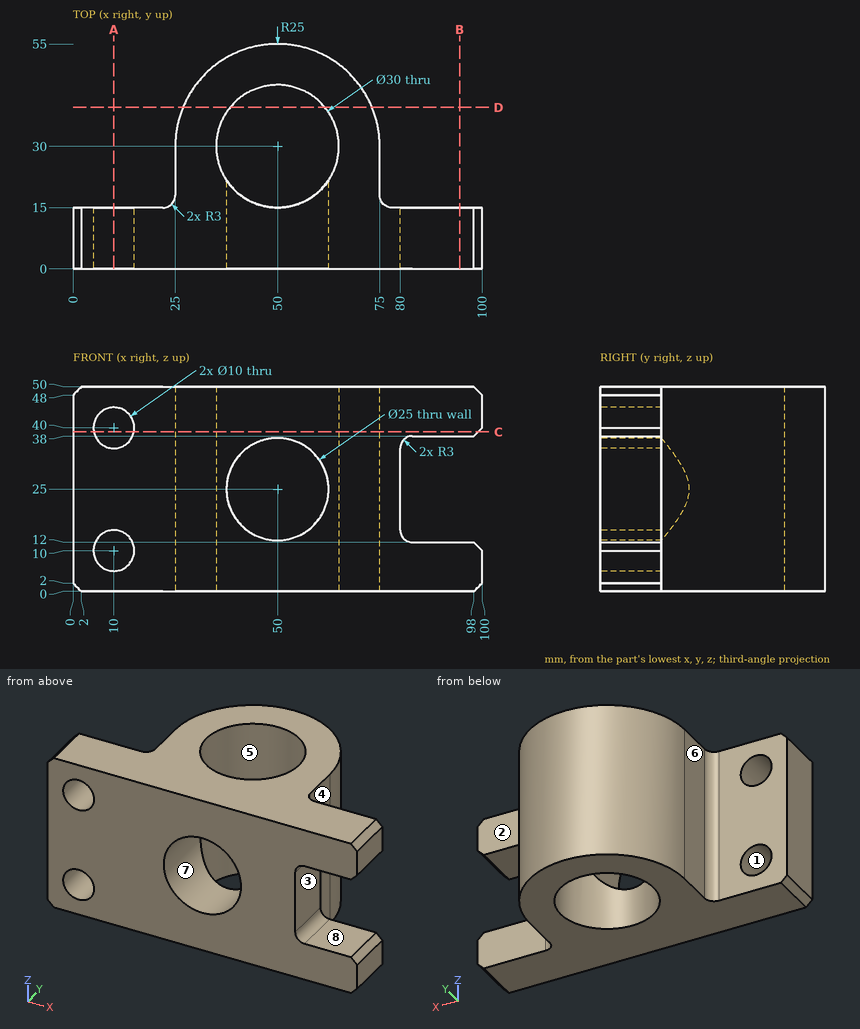
Here's the drawing with two shaded views (mm, measured from the low corner). I have some questions. A direction names the side the tool comes from. Give positions to 0.01 mm unless a question says otherwise; leave off trailing zeros. Loops run counter-clockwise (first coordinate to the right, second up) from the corner with the lowest first, then second, coordinate; pieces in that order, holes last. Notation, with made-up numbers: M 87.5,33 L 99.5,33 A19 cw 99.5,58 Z; hole C 47,76 d1. An arc over 180 degrees is marked long. One line per item, written item: value. Start each with the question number.
1) Thinking about a two-plate mould opening in X: for the marked faces 1, 2 and 3, which applies, +X half, -X half, draft (parallel to the pull), parting line (faces both ways), or undercut?
2) If we section it at B-B, the plane x = 94.5: Write out the boundary of the cut face in (y, z).
3) If we section it at A-A, the plane x = 10: Write out the boundary of the cut face in (y, z).
4) I'm going to push flat-ended pins straight in: pin 1 (2 mm diameter, centred on x = 52.5, z = 15, fed in from -Y); pin 2 (8 mm diameter, centred on x = 28, z = 17.5, fed in from +Y); pin 3 (12 mm diameter, centred on y = 5, z = 21.5, fed in from +X). Where does each tip first touch, or does it pass through?
5) On a 3-axis mill with a long thin cutter (end or side, diameter ignored), from which of +Z, -Z, +X, -X, +Y, -Y can I reach the whole of each face in a straight line? I mean the marked faces 4, 5, 6, 7 and 8. Say none if no direction works.
6) If we section it at D-D, the plane y = 39.5: Write out the boundary of the cut face in (x, z).
7) If we section it at C-C, the plane z = 39: Write out the boundary of the cut face in (x, y), and give its area (3 significant figures).
8) If I drill on line 1 (Z direction, x = 10, y = 4.25); line 2 (Z direction, x = 42.5, y = 12); line 3 (Y direction, x = 16.5, z = 37.5), over which ranges is the centre line in solid material (lowest first)? Write a range as [from, to].
Completed:
1. face 1: undercut
1. face 2: draft
1. face 3: +X half
2. outline: M 0,0 L 15,0 L 15,12 L 0,12 Z; M 0,38 L 15,38 L 15,50 L 0,50 Z
3. outline: M 0,0 L 15,0 L 15,5 L 0,5 Z; M 0,15 L 15,15 L 15,35 L 0,35 Z; M 0,45 L 15,45 L 15,50 L 0,50 Z
4. pin 1: stops at y = 44.59
4. pin 2: stops at y = 47.35
4. pin 3: stops at x = 80
5. face 4: +Z, -Z, +X, +Y
5. face 5: +Z, -Z
5. face 6: +Z, -Z, -X, +Y
5. face 7: -Y
5. face 8: +X, +Y, -Y
6. outline: M 26.88,0 L 38.39,0 L 38.39,50 L 26.88,50 Z; M 61.61,0 L 73.12,0 L 73.12,50 L 61.61,50 Z
7. outline: M 0,0 L 5.1,0 L 5.1,15 L 0,15 Z; M 14.9,0 L 99,0 L 99,15 L 78,15 A3 cw 75,18 L 75,30 A25 ccw 25,30 L 25,18 A3 cw 22,15 L 14.9,15 Z; hole C 50,30 d30
7. area: 2,370 mm^2
8. line 1: z = [0, 5], [15, 35], [45, 50]
8. line 2: z = [0, 15], [35, 50]
8. line 3: y = [0, 15]
